Check sheet for the modelled part. Datum: model origin and axes. Units: mm. Face numbers are marked on the shaded views. A direction names the side the tool comes from. Coordinates: 2 decimals unless noted, no trailing zeros. Write each loop counter-clockwise with the first axis right and the second up, starting at its lowest first coordinate (ties: lowest second). Pieces come first, ordered by that corner, then holes. Notation, with made-up numbers: (-8, 88.5) - (25, 88.5) arc R23 ccw to (25, 109.5) - close; hole circle Ø8 at (80, 82). An arc over 180 degrees is marked (long way). Write each question's results on one line, items separated by ' | '.
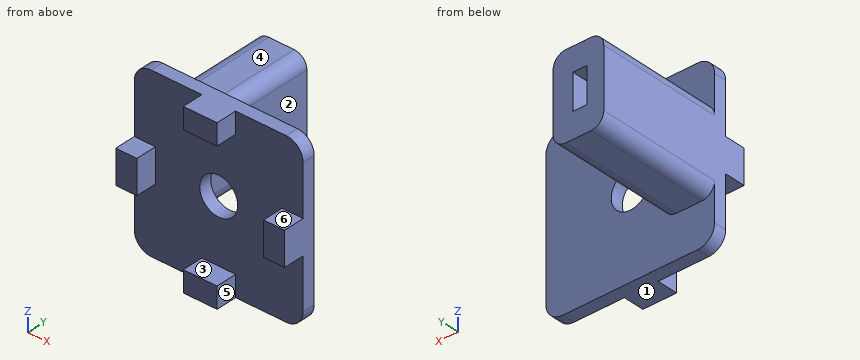
Autodesk Fusion 360 part; units mm, degrees
sketch "Sketch1" plane through (0, 0, 0) normal (0, 1, 0) x (1, 0, 0)
  line L0 (20, -20) -> (-20, -20)
  line L1 (-20, -20) -> (-20, 20)
  line L2 (-20, 20) -> (20, 20)
  line L3 (20, 20) -> (20, -20)
  line L4 (20, -20) -> (-20, 20) construction
  line L5 (-20, -20) -> (20, 20) construction
  line L6 (-20, 4) -> (-15, 4)
  line L7 (-15, 4) -> (-15, -4)
  line L8 (-15, -4) -> (-20, -4)
  line L9 (-20, -4) -> (-20, 4)
  line L10 (-4, 20) -> (4, 20)
  line L11 (4, 20) -> (4, 15)
  line L12 (4, 15) -> (-4, 15)
  line L13 (-4, 15) -> (-4, 20)
  line L14 (20, 4) -> (15, 4)
  line L15 (15, 4) -> (15, -4)
  line L16 (15, -4) -> (20, -4)
  line L17 (20, -4) -> (20, 4)
  line L18 (-4, -20) -> (4, -20)
  line L19 (4, -20) -> (4, -15)
  line L20 (4, -15) -> (-4, -15)
  line L21 (-4, -15) -> (-4, -20)
  dimension "d1" = 40
  dimension "d2" = 40
  dimension "d3" = 5
  dimension "d4" = 8
  dimension "d5" = 16
  dimension "d6" = 5
  dimension "d7" = 16
  dimension "d8" = 8
  dimension "d9" = 5
  dimension "d10" = 5
  dimension "d11" = 8
  dimension "d12" = 8
  dimension "d13" = 16
  dimension "d14" = 16
extrude "Extrude1" add sketch "Sketch1" against normal blind 3 contours L0 L1 L2 L3 L6 L7 L8 L11 L12 L13 L14 L15 L16 L19 L20 L21
extrude "Extrude2" add sketch "Sketch1" against normal blind 8 contours L0 L18 L19 L20 L21 | L3 L14 L15 L16 L17 | L1 L6 L7 L8 L9 | L2 L10 L11 L12 L13
hole "Hole1" at (0, 0, 0) direction (0, -1, 0) diameter 9 depth 30 tip angle 118
fillet "Fillet1" radius 4 4 edges at (20, -1.5, -20) (-20, -1.5, -20) (20, -1.5, 20) (-20, -1.5, 20)
sketch "Sketch2" plane through (0, 0, 0) normal (0, 1, 0) x (1, 0, 0)
  line L0 (-20, 10) -> (-8, 10)
  line L1 (-8, 10) -> (-8, -10)
  line L2 (-8, -10) -> (-20, -10)
  line L3 (-20, -10) -> (-20, 10)
  line L4 (-16, 4) -> (-12.7, 4)
  line L5 (-12.7, 4) -> (-12.7, -4.4)
  line L6 (-12.7, -4.4) -> (-16, -4.4)
  line L7 (-16, -4.4) -> (-16, 4)
  line L8 (-20, 20) -> (20, 20)
  dimension "d24" = 12
  dimension "d25" = 20
  dimension "d26" = 8.4
  dimension "d27" = 3.3
  dimension "d28" = 6
  dimension "d29" = 10
extrude "Extrude3" add sketch "Sketch2" along normal blind 30
fillet "Fillet2" radius 3 4 edges at (-8, 15, 10) (-20, 15, 10) (-8, 15, -10) (-20, 15, -10)
equation "d6 = d3"
equation "d7 = d5"
equation "d8 = d4"
equation "d9 = d3"
equation "d10 = d3"
equation "d11 = d4"
equation "d12 = d4"
equation "d13 = d7"
equation "d14 = d7"
1. Access from +Z, -Z, +X, -X, +Y, -Y to the whole of each face (thin tool, end or side, straight path). Record for the marked faces 4, 5 and 6.
Values follow:
face 4: +Z, +X, -X, +Y | face 5: +Z, -Z, +X, -Y | face 6: +Z, +X, -X, -Y
2. Sectioned sample at C-C (z = 0). Record the cut outline in (x, y), then the cut area to 3 significant figures.
Values follow:
outline: (-20, -8) - (-15, -8) - (-15, -3) - (-4.5, -3) - (-4.5, 0) - (-8, 0) - (-8, 30) - (-12.7, 30) - (-12.7, 0) - (-16, 0) - (-16, 30) - (-20, 30) - close; (4.5, -3) - (15, -3) - (15, -8) - (20, -8) - (20, 0) - (4.5, 0) - close | area: 404 mm^2
3. Material ranges on L1, parallel to X at y = 28, z = -2; L2, parallel to Z at x = 0, y = -1; L3, parallel to Y at x = 2, z = -14.5, recorded low to high. Write a range as [from, to].
Values follow:
L1: x = [-20, -16], [-12.7, -8] | L2: z = [-20, -4.5], [4.5, 20] | L3: y = [-3, 0]
4. Sectioned sample at A-A (x = 0). Record the cut outline in (y, z), then the cut area to 3 significant figures.
Values follow:
outline: (-8, -20) - (0, -20) - (0, -4.5) - (-3, -4.5) - (-3, -15) - (-8, -15) - close; (-8, 15) - (-3, 15) - (-3, 4.5) - (0, 4.5) - (0, 20) - (-8, 20) - close | area: 143 mm^2
5. Go/stop test with flat-tipped pins: pin 1 (8 mm diameter, centred on y = 8.5, z = -0.5, fed in from +X); pin 2 (4 mm diameter, centred on x = -1, z = 14.5, fed in from +Y); pin 3 (5.5 mm diameter, centred on x = 0, z = 0, fed in from +Y); pin 4 (10 mm diameter, centred on x = -15, y = 25.5, fed in from +Z). Record where each tip stops, or that it passes through.
Values follow:
pin 1: stops at x = -8 | pin 2: stops at y = 0 | pin 3: passes through | pin 4: stops at z = 10
6. Sectioned sample at D-D (y = -5). Record the cut outline in (x, z).
Values follow:
outline: (-20, -4) - (-15, -4) - (-15, 4) - (-20, 4) - close; (-4, -20) - (4, -20) - (4, -15) - (-4, -15) - close; (-4, 15) - (4, 15) - (4, 20) - (-4, 20) - close; (15, -4) - (20, -4) - (20, 4) - (15, 4) - close
7. Sectioned sample at B-B (y = 22). Record the cut outline in (x, z), then the cut area to 3 significant figures.
Values follow:
outline: (-20, -7) arc R3 ccw to (-17, -10) - (-11, -10) arc R3 ccw to (-8, -7) - (-8, 7) arc R3 ccw to (-11, 10) - (-17, 10) arc R3 ccw to (-20, 7) - close; hole (-16, -4) - (-12.7, -4) - (-12.7, 4.4) - (-16, 4.4) - close | area: 205 mm^2
8. Draft check along Z on the marked faces 1, 2 and 3. Enter one of: pulls with the +Z half, pulls with the -Z half, needs draft (parallel to the pull), parting line crosses it, or undercut.
Values follow:
face 1: pulls with the -Z half | face 2: needs draft | face 3: undercut
